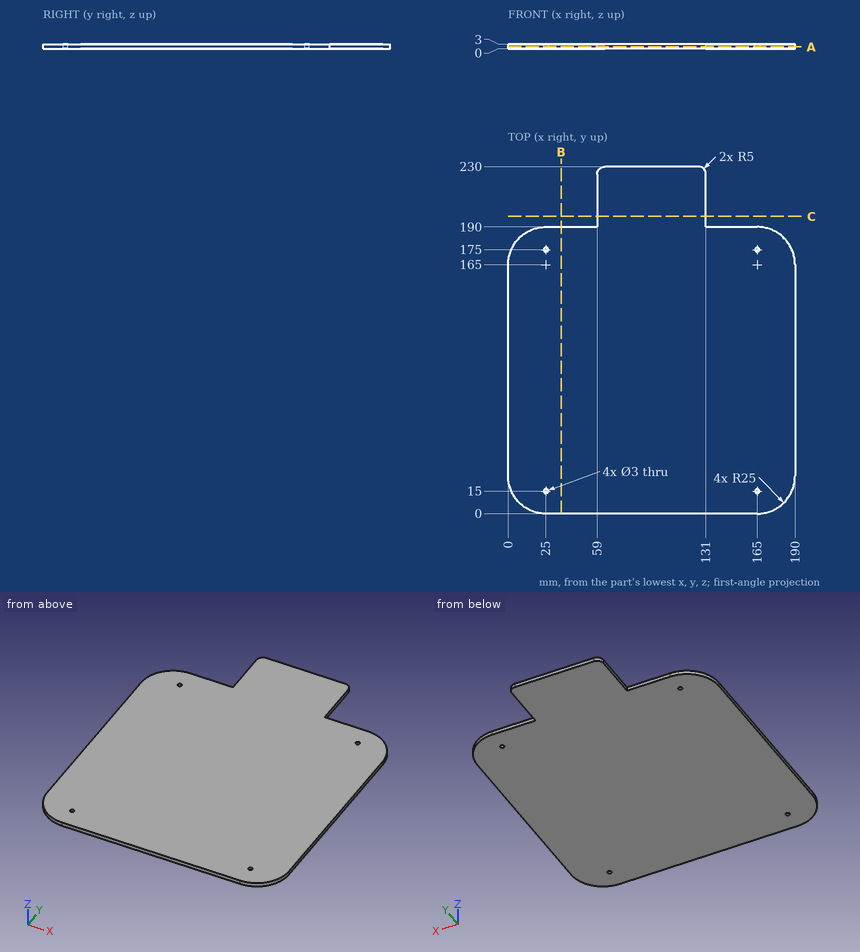
Here's the drawing with two shaded views (mm, measured from the low corner). I have some questions. Give positions to 0.01 mm unless a question says otherwise; leave off trailing zeros. Write each loop counter-clockwise with the first axis right and the second up, starting at its lowest first coordinate (ties: lowest second). Pieces come first, ordered by that corner, then holes. Notation, with made-up numbers: (-32.75, -38) - (-0.75, -38) arc R34 cw to (-0.75, 0) - close; hole circle Ø7 at (-27.5, -22). An arc over 180 degrees is marked (long way). Write item = value, one per line. Start each with the question number.
1. Imagine slicing it at C-C (y = 197). Please give me the cut outline in (x, z), and give its area (3 significant figures).
2. Imagine slicing it at A-A (z = 1.1). Please give me the cut outline in (x, y), and give its area (3 significant figures).
3. Please list where these lines run through material, in increasing order: line 1 (X direction, y = 175, z = 1.2); line 2 (Y direction, x = 46, z = 1.4); line 3 (X direction, y = 205.5, z = 1.4).
4. For pin 1 (0.9 mm diameter, centred on x = 43.5, z = 1.5, fed in from +Y); pin 2 (2.5 mm diameter, centred on x = 165, y = 15, fed in from +Z); pin 3 (0.9 mm diameter, centred on y = 205, z = 1, fed in from +X), each with a flat end and sliding along its axis, tell me the tip position at first contact or that it passes through.
5. Imagine slicing it at B-B (x = 35). Please give me the cut outline in (y, z), and give its area (3 significant figures).
Worked answers:
q1.outline = (59, 0) - (131, 0) - (131, 3) - (59, 3) - close
q1.area = 216 mm2
q2.outline = (0, 25) arc R25 ccw to (25, 0) - (165, 0) arc R25 ccw to (190, 25) - (190, 165) arc R25 ccw to (165, 190) - (131, 190) - (131, 225) arc R5 ccw to (126, 230) - (64, 230) arc R5 ccw to (59, 225) - (59, 190) - (25, 190) arc R25 ccw to (0, 165) - close; hole circle Ø3 at (25, 15); hole circle Ø3 at (25, 175); hole circle Ø3 at (165, 15); hole circle Ø3 at (165, 175)
q2.area = 38,400 mm2
q3.line_1 = 2.09 to 23.5, 26.5 to 163.5, 166.5 to 187.91
q3.line_2 = 0 to 190
q3.line_3 = 59 to 131
q4.pin_1 = 190
q4.pin_2 = through
q4.pin_3 = 131
q5.outline = (0, 0) - (190, 0) - (190, 3) - (0, 3) - close
q5.area = 570 mm2
